Build history of the part. All positions in model axes, mm. A direction names the side the tool comes from. Coordinates: 2 decimals unless noted, no trailing zeros. Write each loop counter-clockwise with the first axis right and the second up, starting at its lowest first coordinate (ties: lowest second). Pieces come first, ordered by that corner, then holes.
```python
from build123d import *
from OCP.BRepFilletAPI import BRepFilletAPI_MakeChamfer

# Parameters (mm, degrees)
DODANIE_WYCI_GNI_CIE1_DEPTH     = 4
DODANIE_WYCI_GNI_CIE2_DEPTH     = 3.2
DODANIE_WYCI_GNI_CIE3_DEPTH     = 4
DODANIE_WYCI_GNI_CIE4_DEPTH     = 32
WYTNIJ_WYCI_GNI_CIE1_DEPTH      = 17.6
WYTNIJ_WYCI_GNI_CIE1_DEPTH_BACK = 17.6
SZKIC5_R                        = 11.1
SFAZOWANIE1_SIZE                = 11.2
SFAZOWANIE1_SIZE_2              = 8
WYTNIJ_WYCI_GNI_CIE2_DEPTH      = 20.2
WYTNIJ_WYCI_GNI_CIE2_DEPTH_BACK = 140.211637445
SZKIC6_R                        = 4.3
SZKIC7_W                        = 4
SZKIC7_H                        = 83
SZKIC7_W_2                      = 3
DODANIE_WYCI_GNI_CIE5_DEPTH     = 32
SFAZOWANIE2_SIZE                = 10
SFAZOWANIE3_SIZE                = 2
SFAZOWANIE3_SIZE2               = 5.494954839
SZKIC8_R                        = 2.1
OTWORY_TYL_DEPTH                = 143.556234518
SZKIC9_R                        = 3.1
SZKIC9_R_2                      = 2.1
OTWORY_SPOD_DEPTH               = 148.729482501
SZKIC10_R                       = 2.1
OTWORY_BOK_DEPTH                = 146.390095949
SFAZOWANIE4_SIZE                = 8
SZKIC11_W                       = 89.626948643
SZKIC11_H                       = 50.587454561
WYTNIJ_WYCI_GNI_CIE3_DEPTH      = 158.003948995


with BuildPart() as part:
    # Szkic1 → Dodanie-wyciągnięcie1 (new body)
    with BuildSketch(Plane.XY):
        Polygon((0, 0), (80, 0), (20, -120), (0, -120), align=None)
    extrude(amount=DODANIE_WYCI_GNI_CIE1_DEPTH)

    # Szkic2 → Dodanie-wyciągnięcie2 (add)
    with BuildSketch(Plane.XY.offset(4)):
        Polygon((80, 0), (0, 0), (0, -120), (4, -120), (4, -4), (78, -4), align=None)
    extrude(amount=DODANIE_WYCI_GNI_CIE2_DEPTH)

    # Szkic3 → Dodanie-wyciągnięcie3 (add)
    with BuildSketch(Plane.XY.offset(7.2)):
        Polygon((78, -4), (80, 0), (0, 0), (0, -120), (4, -120), (20, -120), align=None)
    extrude(amount=DODANIE_WYCI_GNI_CIE3_DEPTH)

    # Szkic4 → Dodanie-wyciągnięcie4 (add)
    with BuildSketch(Plane.XY.offset(11.2)):
        Polygon((0, 8), (0, -37), (48.4, -37), (48.4, 8), (34.4, 8), (34.4, -24), (14, -24), (14, 8), align=None)
    extrude(amount=DODANIE_WYCI_GNI_CIE4_DEPTH)

    # Szkic5 → Wytnij-wyciągnięcie1 (cut, two sides: drawn at the far end of the back side and taken through both)
    with BuildSketch(Plane(origin=(24.2, 0, 0), x_dir=(0, 0, -1), z_dir=(1, 0, 0)).offset(-WYTNIJ_WYCI_GNI_CIE1_DEPTH_BACK)):
        with Locations(Location((-27.2, -8, 0), (0, 0, 180))):
            Circle(SZKIC5_R)
    extrude(amount=WYTNIJ_WYCI_GNI_CIE1_DEPTH + WYTNIJ_WYCI_GNI_CIE1_DEPTH_BACK, mode=Mode.SUBTRACT)

    # Sfazowanie1
    sfazowanie1_edges_1 = [part.edges().sort_by_distance(p)[0] for p in [
        (7, 0, 11.2),
    ]]
    sfazowanie1_side_1 = [part.faces().sort_by_distance(p)[0] for p in [
        (7, 0, 11.04),
    ]]
    sfazowanie1_edges_2 = [part.edges().sort_by_distance(p)[0] for p in [
        (41.4, 0, 11.2),
    ]]
    sfazowanie1_side_2 = [part.faces().sort_by_distance(p)[0] for p in [
        (41.4, 0, 11.04),
    ]]
    sfazowanie1 = BRepFilletAPI_MakeChamfer(part.part.solid().wrapped)
    for e in sfazowanie1_edges_1:
        sfazowanie1.Add(SFAZOWANIE1_SIZE - 0.0001, SFAZOWANIE1_SIZE_2 - 0.0001, e.wrapped, sfazowanie1_side_1[0].wrapped)
    for e in sfazowanie1_edges_2:
        sfazowanie1.Add(SFAZOWANIE1_SIZE - 0.0001, SFAZOWANIE1_SIZE_2 - 0.0001, e.wrapped, sfazowanie1_side_2[0].wrapped)
    add(Compound.cast(sfazowanie1.Shape()), mode=Mode.REPLACE)  # a hair under: the kernel refuses the full size

    # Szkic6 → Wytnij-wyciągnięcie2 (cut, two sides: drawn at the far end of the back side and taken through both)
    with BuildSketch(Plane(origin=(24.2, 0, 0), x_dir=(0, 0, -1), z_dir=(1, 0, 0)).offset(-WYTNIJ_WYCI_GNI_CIE2_DEPTH_BACK)):
        with Locations((-27.2, -8)):
            Circle(SZKIC6_R)
    extrude(amount=WYTNIJ_WYCI_GNI_CIE2_DEPTH + WYTNIJ_WYCI_GNI_CIE2_DEPTH_BACK, mode=Mode.SUBTRACT)

    # Szkic7 → Dodanie-wyciągnięcie5 (add)
    with BuildSketch(Plane.XY.offset(11.2)):
        with Locations((2, -78.5)):
            Rectangle(SZKIC7_W, SZKIC7_H)
        with Locations((8.7, -78.5)):
            Rectangle(SZKIC7_W_2, SZKIC7_H)
        Polygon((48.4, 0), (80, 0), (78, -4), (48.4, -4), align=None)
        Polygon((48.4, -7.2), (76.4, -7.2), (74.9, -10.2), (48.4, -10.2), align=None)
    extrude(amount=DODANIE_WYCI_GNI_CIE5_DEPTH)

    # Sfazowanie2
    sfazowanie2_edges = [part.edges().sort_by_distance(p)[0] for p in [
        (10.2, -37, 27.2),
        (48.4, -10.2, 27.2),
        (48.4, -37, 27.2),
    ]]
    chamfer(sfazowanie2_edges, length=SFAZOWANIE2_SIZE)

    # Sfazowanie3
    sfazowanie3_edges = [part.edges().sort_by_distance(p)[0] for p in [
        (10.2, -83.5, 11.2),
        (48.4, -23.6, 11.2),
        (29.3, -37, 11.2),
        (66.65, -10.2, 11.2),
        (15.2, -42, 11.2),
        (53.4, -15.2, 11.2),
        (43.4, -32, 11.2),
    ]]
    sfazowanie3_side = [part.faces().sort_by_distance(p)[0] for p in [
        (33.378295522, -61.643653627, 11.2),
    ]]
    chamfer(sfazowanie3_edges, length=SFAZOWANIE3_SIZE, length2=SFAZOWANIE3_SIZE2, reference=sfazowanie3_side[0])

    # Szkic8 → Otwory tyl (cut, through all)
    with BuildSketch(Plane.XZ.offset(10.2)):
        with Locations((66.65, 35.2)):
            Circle(SZKIC8_R)
        with Locations((66.65, 21.2)):
            Circle(SZKIC8_R)
    extrude(amount=-OTWORY_TYL_DEPTH, mode=Mode.SUBTRACT)

    # Szkic9 → Otwory spod (cut, through all)
    with BuildSketch(Plane.XY.offset(11.2)):
        with Locations((60.4, -22.2)):
            Circle(SZKIC9_R)
        with Locations((22.2, -49)):
            Circle(SZKIC9_R_2)
        with Locations((22.2, -89)):
            Circle(SZKIC9_R_2)
        with Locations((36.2, -49)):
            Circle(SZKIC9_R_2)
    extrude(amount=-OTWORY_SPOD_DEPTH, mode=Mode.SUBTRACT)

    # Szkic10 → Otwory bok (cut, through all)
    with BuildSketch(Plane(origin=(10.2, 0, 0), x_dir=(0, 0, -1), z_dir=(1, 0, 0))):
        with Locations(Location((-23.2, -80, 0), (0, 0, 90))):
            Circle(SZKIC10_R)
        with Locations(Location((-35.2, -55, 0), (0, 0, 90))):
            Circle(SZKIC10_R)
        with Locations(Location((-23.2, -105, 0), (0, 0, 90))):
            Circle(SZKIC10_R)
    extrude(amount=-OTWORY_BOK_DEPTH, mode=Mode.SUBTRACT)

    # Sfazowanie4
    sfazowanie4_edges = [part.edges().sort_by_distance(p)[0] for p in [
        (48.4, 0, 21.60005),
    ]]
    chamfer(sfazowanie4_edges, length=SFAZOWANIE4_SIZE - 0.0001)  # a hair under: the kernel refuses the full size


with BuildPart() as body_2:
    # Lustro1: mirrored copy
    add(part.part.mirror(Plane(origin=(0, 0, 4), x_dir=(0, 0, 1), z_dir=(1, 0, 0))))


with BuildPart() as part_1:
    add(part.part)

    # Szkic11 → Wytnij-wyciągnięcie3 (cut, through all)
    with BuildSketch(Plane.XZ.offset(120)):
        with Locations((44.813474322, 25.293727281)):
            Rectangle(SZKIC11_W, SZKIC11_H)
    extrude(amount=-WYTNIJ_WYCI_GNI_CIE3_DEPTH, mode=Mode.SUBTRACT)


solid = body_2.part
```
1. 3-axis set-ups, long thin cutter, end or side, ignore diameter. For faces 5 (the face through (-40, -4, 6)), 6 (the face through (-7.2, -79, 27)), 7 (the face through (-63, -4, 27)), 8 (the face through (-6.6, -8, 32)), 9 (the face through (-10.2, -84, 30)): which of +Z, -Z, +X, -X, +Y, -Y reach the whole face in a straight line?
Computed values:
face 5: -X, -Y
face 6: +Z, -Y
face 7: +Z, -X
face 8: none
face 9: +Z, -X, -Y
2. Saw through at C-C on y = -16. List the corners of the cut face in (x, z).
Computed values:
outline: (-72, 0) - (0, 0) - (0, 43.2) - (-14, 43.2) - (-14, 34.89) - (-6.6, 34.89) - (-6.6, 19.51) - (-14, 19.51) - (-14, 11.2) - (-34.4, 11.2) - (-34.4, 19.51) - (-41.8, 19.51) - (-41.8, 34.89) - (-34.4, 34.89) - (-34.4, 43.2) - (-52.6, 43.2) - (-52.6, 16.69) - (-55.43, 11.2) - (-72, 11.2) - (-72, 7.2) - (-4, 7.2) - (-4, 4) - (-72, 4) - close
3. Probe line 1 along Z through (x, y) = (-43.05, -8); line 2 along Z through (x, y) = (-39, -75); line 3 along Z through (x, y) = (-1.3, -55). List the from-to ranges inside material, lowest first.
Computed values:
line 1: z = 0 to 4, 7.2 to 22.9, 31.5 to 43.2
line 2: z = 0 to 4, 7.2 to 11.2
line 3: z = 0 to 33.1, 37.3 to 43.2
4. Mould opens along X. For faces 1 (the face through (-64.55, -2.03, 21.29)), 2 (the face through (-20.534, -90.278, 9.228)), 3 (the face through (-49.386, -24.068, 13.986)), 4 (the face through (-29, -37, 30)) say: +X half, -X half, draft (parallel to the pull), parting line (faces both ways), or undercut.
Computed values:
face 1: undercut
face 2: undercut
face 3: -X half
face 4: draft
5. Flat gauge pins, fed straight in: pin 1 (5.5 mm diameter, centred on y = -105, z = 23.2, fed in from -X); pin 2 (12 mm diameter, centred on x = -22, z = 37.5, fed in from -Y); pin 3 (2 mm diameter, centred on x = -40.5, z = 16.5, fed in from -Y); pin 4 (4 mm diameter, centred on x = -66.65, z = 21.2, fed in from +Y) (3 decimals). Where does each tip first touch, or does it go through?
Computed values:
pin 1: stops at x = -10.2
pin 2: stops at y = -41.2
pin 3: stops at y = -36.13
pin 4: passes through
6. Saw through at B-B on x = -32. List the corners of the cut face in (y, z), plus the area to 3 significant figures.
Computed values:
outline: (-96, 0) - (0, 0) - (0, 11.2) - (-24, 11.2) - (-24, 43.2) - (-37, 43.2) - (-37, 16.69) - (-39, 11.2) - (-96, 11.2) - (-96, 7.2) - (-4, 7.2) - (-4, 4) - (-96, 4) - close
area: 1,200 mm2
7. Saw through at A-A on y = -89. List the corners of the cut face in (x, z), plus the area to 3 significant figures.
Computed values:
outline: (-35.5, 0) - (-24.3, 0) - (-24.3, 4) - (-35.5, 4) - close; (-35.5, 7.2) - (-24.3, 7.2) - (-24.3, 11.2) - (-35.5, 11.2) - close; (-20.1, 0) - (0, 0) - (0, 43.2) - (-4, 43.2) - (-4, 11.2) - (-7.2, 11.2) - (-7.2, 43.2) - (-10.2, 43.2) - (-10.2, 16.69) - (-12.2, 11.2) - (-20.1, 11.2) - (-20.1, 7.2) - (-4, 7.2) - (-4, 4) - (-20.1, 4) - close
area: 493 mm2
